Geometry: final body of the model. Coordinates: model frame, mm. Face numbers are marked on the shaded views. A direction names the side the tool comes from. Round coordinates to 2 decimals unless told otherwise and drop trailing zeros. Loops run counter-clockwise (first coordinate to the right, second up) from the corner with the lowest first, then second, coordinate; pieces in that order, holes last. Notation, with made-up numbers: (-10, -36) - (40, -36) arc R27 ccw to (40, -12) - close; hole circle Ø4 at (23, 55). An arc over 180 degrees is marked (long way). Use CSV: the item, a comma, the result in double quotes.
from build123d import *

# Parameters (mm, degrees)
SKETCH1_R      = 2.5
EXTRUDE1_DEPTH = 0.5
SKETCH2_R      = 0.75
EXTRUDE2_DEPTH = 25
CHAMFER1_SIZE  = 2
CHAMFER1_SIZE2 = 0.7


with BuildPart() as part:
    # Sketch1 → Extrude1 (new body)
    with BuildSketch(Plane.XY):
        Circle(SKETCH1_R)
    extrude(amount=EXTRUDE1_DEPTH)

    # Sketch2 → Extrude2 (add)
    with BuildSketch(Plane.XY.offset(0.5)):
        Circle(SKETCH2_R)
    extrude(amount=EXTRUDE2_DEPTH)

    # Chamfer1
    chamfer1_edges = [part.edges().sort_by_distance(p)[0] for p in [
        (-0.75, 0, 25.5),
    ]]
    chamfer1_side = [part.faces().sort_by_distance(p)[0] for p in [
        (-0.75, 0, 13),
    ]]
    chamfer(chamfer1_edges, length=CHAMFER1_SIZE, length2=CHAMFER1_SIZE2, reference=chamfer1_side[0])


solid = part.part
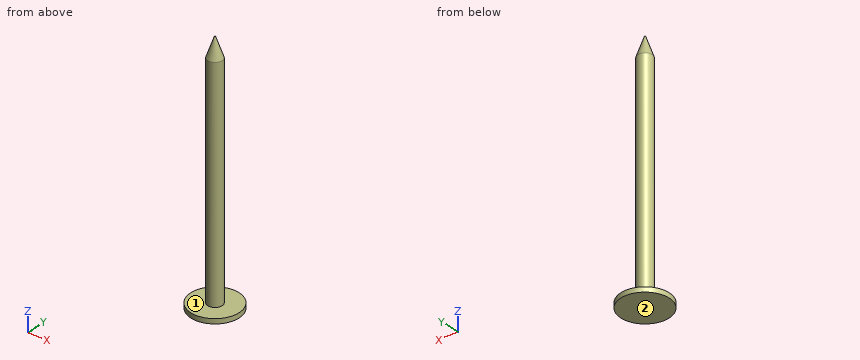
Item 1: Section A-A on z = 23. Return the cut outline in (x, y).
Final values:
outline,"circle Ø1.5 at (0, 0)"
Item 2: Pin query (flat end, axial travel): P1, Ø3, axis at x = 1, z = 7, coming from the -Y side. Return the tip coordinate at first contact, or that it passes through.
Final values:
P1,"stops at y = -0.75"
Item 3: Material intervals for line 1 (Z direction, x = 1.25, y = -0.85); line 2 (Y direction, x = 0.4, z = 5.5); line 3 (X direction, y = 0.5, z = 18.25), sorted ascending.
Final values:
line 1,"z = 0 to 0.5"
line 2,"y = -0.63 to 0.63"
line 3,"x = -0.56 to 0.56"
Item 4: Section C-C on y = -1.4. Return the cut outline in (x, z).
Final values:
outline,"(-2.07, 0) - (2.07, 0) - (2.07, 0.5) - (-2.07, 0.5) - close"
Item 5: Section B-B on x = 2. Return the cut outline in (y, z).
Final values:
outline,"(-1.5, 0) - (1.5, 0) - (1.5, 0.5) - (-1.5, 0.5) - close"
Item 6: Reachability of the marked faces 1 and 2 from +Z, -Z, +X, -X, +Y, -Y: full face, straight path, thin tool, end or side. Return the list, or none.
Final values:
face 1,"+Z"
face 2,"-Z, +X, -X, +Y, -Y"
